Input: part model. Units: mm. Frame: model coordinates. A direction names the side the tool comes from. Round coordinates to 2 decimals unless told otherwise and drop trailing zeros. Loops run counter-clockwise (first coordinate to the right, second up) from the corner with the lowest first, then second, coordinate; pieces in that order, holes last. Notation, with made-up numbers: M 40.25,0.25 L 80.25,0.25 A24 ccw 80.25,39.25 Z; hole C 7.5,-40 d8. An arc over 180 degrees is marked long. Return JSON: item names as keys, results as strings. Group by question number.
1) Section B-B (z = 28). Output: boundary loops of the cut face in (x, y).
2) Contact query for flat-ended pins moving along their axis: P1, Ø9.5, axis at y = -15.5, z = 22, coming from the -X side; P2, Ø1, axis at x = 11.5, y = -21, coming from the +Z side; P3, Ø6.5, axis at x = 9.5, y = -15, coming from the +Z side. Output: stop coordinate, or through.
3) Material intervals for line 1 (Y direction, x = 16.75, z = 28); line 2 (Z direction, x = 1, y = -34); line 3 (X direction, y = -20.5, z = 16.5), sorted ascending. Write a range as from..to.
4) Section A-A (x = 23.25). Output: boundary loops of the cut face in (y, z).
5) Section C-C (y = -21). Output: boundary loops of the cut face in (x, z).
6) Access query for faces 1 (the face through (19, -25.4, 28)), 2 (the face through (6, -19, 12.7)), 3 (the face through (19, -6, 31.75)). Directions: +Z, -Z, +X, -X, +Y, -Y. A direction counts if a zero-diameter tool reaches every point of the face in a straight line with its end or side. Return the directions, or none.
7) Section D-D (z = 23). Output: boundary loops of the cut face in (x, y), plus the area to 3 significant figures.
from build123d import *

# Parameters (mm, degrees)
F0_W     = 38.1
F0_H     = 31.75
F1_DEPTH = 25.4
F2_W     = 12.7
F2_H     = 19.05
F3_DEPTH = 38.1
F4_W     = 12.7
F4_H     = 7.042224
F5_DEPTH = 25.4


with BuildPart() as f1:
    # F0 (on Right) → F1 (new body)
    with BuildSketch(Plane.YZ):
        with Locations((-19.05, 15.875)):
            Rectangle(F0_W, F0_H)
    extrude(amount=F1_DEPTH)

    # F2 (on face) → F3 (cut)
    with BuildSketch(Plane.XZ.offset(38.1)):
        with Locations((6.35, 22.225)):
            Rectangle(F2_W, F2_H)
    extrude(amount=-F3_DEPTH, mode=Mode.SUBTRACT)

    # F4 (on face) → F5 (cut)
    with BuildSketch(Plane(origin=(12.7, 0, 0), x_dir=(0, -1, 0), z_dir=(-1, 0, 0))):
        with Locations((19.05, 28.228888)):
            Rectangle(F4_W, F4_H)
    extrude(amount=-F5_DEPTH, mode=Mode.SUBTRACT)


solid = f1.part
Returned:
{
 "1": {"outline": "M 12.7,-38.1 L 25.4,-38.1 L 25.4,-25.4 L 12.7,-25.4 Z; M 12.7,-12.7 L 25.4,-12.7 L 25.4,0 L 12.7,0 Z"},
 "2": {"P1": "stops at x = 12.7", "P2": "stops at z = 12.7", "P3": "stops at z = 24.71"},
 "3": {"line 1": "y = -38.1..-25.4, -12.7..0", "line 2": "z = 0..12.7", "line 3": "x = 12.7..25.4"},
 "4": {"outline": "M -38.1,0 L 0,0 L 0,31.75 L -12.7,31.75 L -12.7,24.71 L -25.4,24.71 L -25.4,31.75 L -38.1,31.75 Z"},
 "5": {"outline": "M 0,0 L 25.4,0 L 25.4,24.71 L 12.7,24.71 L 12.7,12.7 L 0,12.7 Z"},
 "6": {"face 1": "+Z, +X, -X", "face 2": "+Z, -X, +Y, -Y", "face 3": "+Z, +X, -X, +Y, -Y"},
 "7": {"outline": "M 12.7,-38.1 L 25.4,-38.1 L 25.4,0 L 12.7,0 Z", "area": "484 mm^2"}
}
